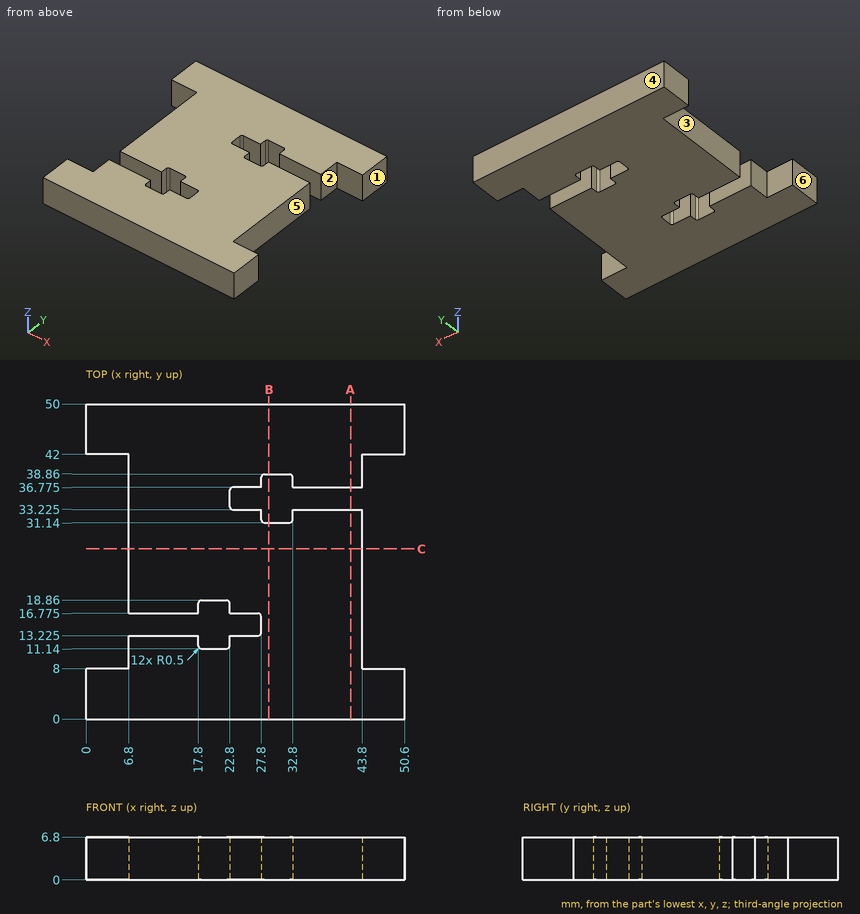
Check sheet for the drawn part. Datum: minimum x, y, z corner. Units: mm. A direction names the side the tool comes from. Coordinates: 2 decimals unless noted, no trailing zeros. Order: outer loops, then holes, each group sorted by start corner. A loop starts at its lowest first (then second) coordinate and runs counter-clockwise, first axis right, second up. Notation, with made-up numbers: M 11.25,40 L 44.25,40 A8 cw 44.25,49 Z; hole C 89,41 d1. An arc over 180 degrees is marked long. One line per item, written item: value. Start each with the question number.
Item 1: Sectioned sample at B-B (x = 29). Enter the section's corners in (y, z).
Item 2: Access from +Z, -Z, +X, -X, +Y, -Y to the whole of each face (thin tool, end or side, straight path). Record for the marked faces 1, 2 and 3.
Item 3: Mould release check, pull along Y, two halves, no side actions. Record for the marked faces 4, 5 and 6: released by +Y, released by -Y, zero draft, split by the parting line, or undercut.
Item 4: Sectioned sample at A-A (x = 42). Enter the section's corners in (y, z) (3 decimals), then the cut area to 3 significant figures.
Item 5: Scan lines: probe 1 along Y at (x, z) = (25, 4) (3 decimals); probe 2 along Y at (x, z) = (12.5, 1.5) (3 decimals); probe 3 along Y at (x, z) = (30, 3.25). Record each from-to range of solid material in increasing order.
Item 6: Gauge pin test, flat ends, axial feed: pin 1 (2 mm diameter, centred on y = 22, z = 2, fed in from +X); pin 2 (1.7 mm diameter, centred on y = 37.5, z = 3.5, fed in from -X). Record the tip position at first contact, or that the pin passes through.
Item 7: Sectioned sample at C-C (y = 27). Enter the section's corners in (x, z).
Conclusion:
1. outline: M 0,0 L 31.14,0 L 31.14,6.8 L 0,6.8 Z; M 38.86,0 L 50,0 L 50,6.8 L 38.86,6.8 Z
2. face 1: +Z, -Z, +X, +Y, -Y
2. face 2: +Z, -Z, +X
2. face 3: +Z, -Z, -X
3. face 4: released by +Y
3. face 5: undercut
3. face 6: zero draft
4. outline: M 0,0 L 33.225,0 L 33.225,6.8 L 0,6.8 Z; M 36.775,0 L 50,0 L 50,6.8 L 36.775,6.8 Z
4. area: 316 mm^2
5. probe 1: y = 0 to 13.225, 16.775 to 33.225, 36.775 to 50
5. probe 2: y = 0 to 13.225, 16.775 to 50
5. probe 3: y = 0 to 31.14, 38.86 to 50
6. pin 1: stops at x = 43.8
6. pin 2: stops at x = 6.8
7. outline: M 6.8,0 L 43.8,0 L 43.8,6.8 L 6.8,6.8 Z
